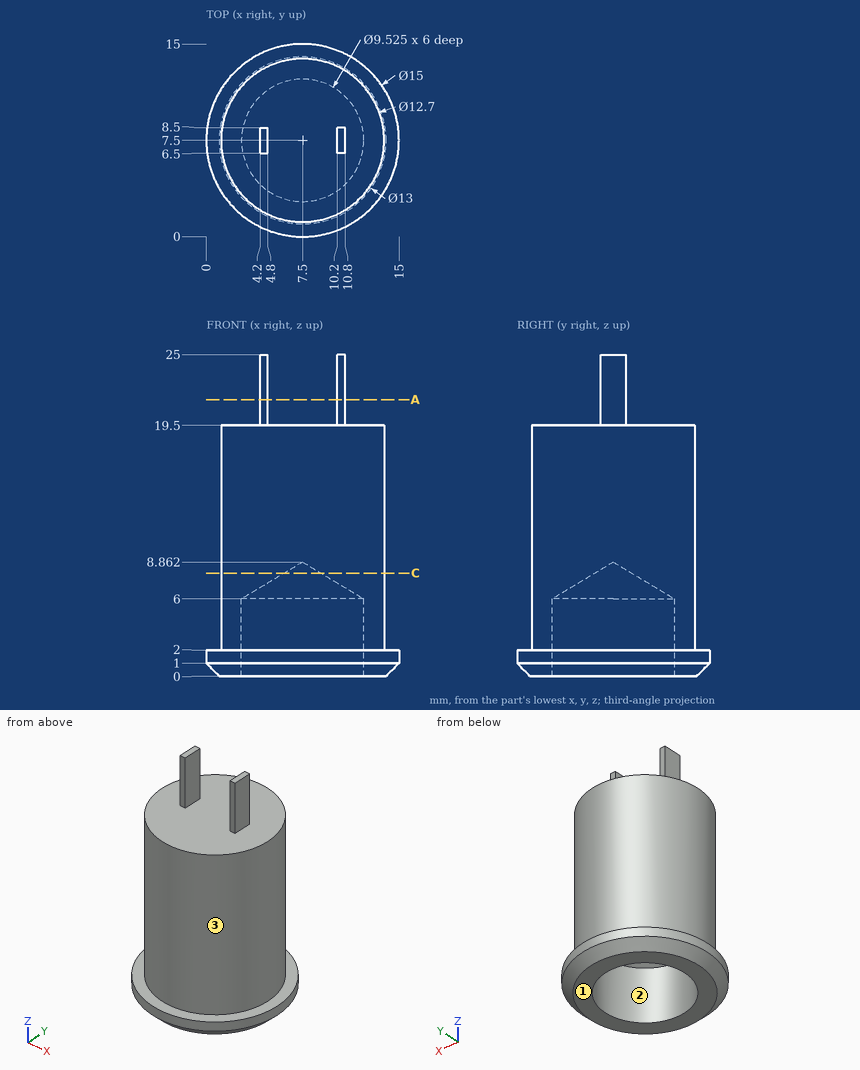
Source: three-view drawing plus pictorial views. Frame: mm from the lowest corner of the part. Coordinates: 2 decimals unless noted, no trailing zeros. Order: outer loops, then holes, each group sorted by start corner. A loop starts at its lowest first (then second) coordinate and runs counter-clockwise, first axis right, second up. Notation, with made-up numbers: M 1.25,84 L 40.25,84 A30 cw 40.25,118 Z; hole C 2.25,38.25 d7. An arc over 180 degrees is marked long. One line per question, with ' | ' between items. Start each with the question number.
Item 1: Cut plane C-C, the plane z = 8. Return the cut outline in (x, y), then the cut area to 3 significant figures.
Item 2: Ray query, probe 1 along Y at (x, z) = (7.5, 4.7); probe 2 along Z at (x, y) = (3.25, 12); probe 3 along Y at (x, z) = (7.5, 18.5). Return the intervals inside material, ascending. Write a range as [from, to].
Item 3: Cut plane A-A, the plane z = 21.5. Return the cut outline in (x, y).
Item 4: Pin query (flat end, axial travel): pin 1 Ø0.7 at (x, z) = (10.5, 23.5) entering from -Y; pin 2 Ø2 at (y, z) = (7.5, 22.5) entering from +X; pin 3 Ø3 at (x, z) = (6.5, 14.5) entering from -Y. Return the tip coordinate at first contact, or that it passes through.
Item 5: Draft query along X for the marked faces 1, 2 and 3. Return one class per face: released by +X, released by -X, zero draft, split by the parting line, or undercut.
A:
1) outline: C 7.5,7.5 d12.7; hole C 7.5,7.5 d2.87 | area: 120 mm2
2) probe 1: y = [1.15, 2.74], [12.26, 13.85] | probe 2: z = [0, 19.5] | probe 3: y = [1.15, 13.85]
3) outline: M 4.2,6.5 L 4.8,6.5 L 4.8,8.5 L 4.2,8.5 Z; M 10.2,6.5 L 10.8,6.5 L 10.8,8.5 L 10.2,8.5 Z
4) pin 1: stops at y = 6.5 | pin 2: stops at x = 10.8 | pin 3: stops at y = 1.15
5) face 1: zero draft | face 2: undercut | face 3: split by the parting line
